CAD build for the part. Positions are in the model's coordinates, mm. A direction names the side the tool comes from. Give positions to 0.01 mm unless a question says otherwise; leave off trailing zeros. Write each loop counter-clockwise with the first axis right and the second up, starting at its lowest first coordinate (ties: lowest second). Pieces come first, ordered by that corner, then holes. Notation, with made-up numbers: (-26, -21) - (21, -21) arc R27 ccw to (21, 10) - close; hole circle Ø1 at (50, 48). An arc over 180 degrees is marked (long way). Answer as a JSON object with one key per item and string values.
Autodesk Inventor part; units mm, degrees
ref_plane "YZ Plane" through (0, 0, 0) normal (1, 0, 0) x (0, 1, 0)
ref_plane "XZ Plane" through (0, 0, 0) normal (0, 1, 0) x (-1, 0, 0)
ref_plane "XY Plane" through (0, 0, 0) normal (0, 0, 1) x (1, 0, 0)
sketch "Sketch1" plane through (0, 0, 0) normal (0, 1, 0) x (-1, 0, 0)
  point P0 (0, 0)
sketch "Sketch2" plane through (0, 0, 0) normal (0, 1, 0) x (-1, 0, 0)
  line L0 (-50, 50) -> (50, 50)
  line L1 (50, 50) -> (50, -50)
  line L2 (50, -50) -> (-50, -50)
  line L3 (-50, -50) -> (-50, 50)
  line L4 (-50, 50) -> (50, -50) construction
  line L5 (50, 50) -> (-50, -50) construction
  point P0 (0, 0)
  dimension "d0" = 100
  dimension "d1" = 100
extrude "Extrusion1" add sketch "Sketch2" against normal blind 50
sketch "Sketch3" plane through (0, 0, 0) normal (0, 1, 0) x (1, 0, 0)
  circle A0 centre (0, 0) radius 30
  dimension "d4" = 60
extrude "Extrusion2" add sketch "Sketch3" along normal blind 50
sketch "Sketch4" plane through (0, 50, 0) normal (0, 1, 0) x (1, 0, 0)
  point P0 (0, 0)
hole "Hole1" at (0, 50, 0) direction (0, -1, 0) diameter 45 depth 30
thread "Thread1"
fillet "Fillet1" radius 3 1 edges at (-30, 50, 0)
sketch "Sketch9" plane through (0, 0, 0) normal (0, 1, 0) x (1, 0, 0)
  circle A0 centre (45, 45) radius 4
  circle A1 centre (45, 45) radius 5
  circle A2 centre (45, -45) radius 5
  circle A3 centre (45, -45) radius 4
  circle A4 centre (-45, 45) radius 4
  circle A5 centre (-45, 45) radius 5
  circle A6 centre (-45, -45) radius 4
  circle A7 centre (-45, -45) radius 5
  point P0 (0, 0)
  point P1 (-50, 50)
  point P2 (-50, -50)
fillet "Fillet6" radius 5 1 edges at (-50, -25, 50)
fillet "Fillet7" radius 5 1 edges at (-50, -25, -50)
fillet "Fillet8" radius 5 1 edges at (50, -25, -50)
fillet "Fillet9" radius 5 1 edges at (50, -25, 50)
hole "Hole7" at (45, 0, -45) direction (0, -1, 0) diameter 8 end through all
hole "Hole8" at (45, 0, 45) direction (0, -1, 0) diameter 8 end through all
hole "Hole9" at (-45, 0, 45) direction (0, -1, 0) diameter 8 end through all
hole "Hole10" at (-45, 0, -45) direction (0, -1, 0) diameter 8 end through all
properties part number "Practica1 - Jonnathan Lanuza"
Item 1: Flat gauge pins, fed straight in: P1, Ø8, axis at x = -29, y = 21.5, coming from the -Z side; P2, Ø4, axis at x = 4, y = 38.5, coming from the -Z side; P3, Ø13.5, axis at x = -2, z = 1.5, coming from the +Y side. Where does each tip first touch, or does it go through?
Entries:
{"P1": "z = -16.58", "P2": "z = -29.93", "P3": "y = 20"}
Item 2: Mould opens along Z. For faces 1 (the flat face through (0, 20, 0)), 2 (the cylindrical face through (-49, -25, -48)), 3 (the cylindrical face through (-29.97, 23.17, 1.32)) say: +Z half, -Z half, draft (parallel to the pull), parting line (faces both ways), or undercut.
Entries:
{"face 1": "undercut", "face 2": "-Z half", "face 3": "parting line"}
Item 3: Which spindle directions (+Z, -Z, +X, -X, +Y, -Y) get a long thin tool onto all of the face, cutting with end or side? Do faces 4 (the cylindrical face through (48, -25, -49)), 5 (the flat face through (23, 0, 23)). Say none if no direction does.
Entries:
{"face 4": "-Z, +X, +Y, -Y", "face 5": "+Y"}
Item 4: Cut at A-A (z = 0). Give the cut face in (x, y).
Entries:
{"outline": "(-50, -50) - (50, -50) - (50, 0) - (30, 0) - (30, 47) arc R3 ccw to (27, 50) - (22.5, 50) - (22.5, 20) - (-22.5, 20) - (-22.5, 50) - (-27, 50) arc R3 ccw to (-30, 47) - (-30, 0) - (-50, 0) - close"}
Item 5: Cut at B-B (x = 0). Give the cut face in (y, z), and give its area (3 significant figures).
Entries:
{"outline": "(-50, -50) - (0, -50) - (0, -30) - (47, -30) arc R3 ccw to (50, -27) - (50, -22.5) - (20, -22.5) - (20, 22.5) - (50, 22.5) - (50, 27) arc R3 ccw to (47, 30) - (0, 30) - (0, 50) - (-50, 50) - close", "area": "6,650 mm2"}
Item 6: Probe line 1 (Z direction, x = 45, y = -34); line 2 (X direction, y = 37.5, z = 0). List the from-to ranges inside material, lowest first. Write a range as from..to.
Entries:
{"line 1": "-50..-49, -41..41, 49..50", "line 2": "-30..-22.5, 22.5..30"}
Item 7: Cut at C-C (y = 27). Give the cut face in (x, z), and give its area (3 significant figures).
Entries:
{"outline": "circle Ø60 at (0, 0); hole circle Ø45 at (0, 0)", "area": "1,240 mm2"}
